Check sheet for the modelled part. Datum: model origin and axes. Units: mm. Face numbers are marked on the shaded views. Coordinates: 2 decimals unless noted, no trailing zeros. Write each loop counter-clockwise with the first axis right and the second up, starting at its lowest first coordinate (ties: lowest second). Pieces come first, ordered by that corner, then holes. Notation, with made-up numbers: (81.25, 41.25) - (110.25, 41.25) arc R23 ccw to (110.25, 68.25) - close; hole circle Ø2 at (70, 38). An arc over 180 degrees is marked (long way). Answer as CSV lines item,"result". Start each with the question number.
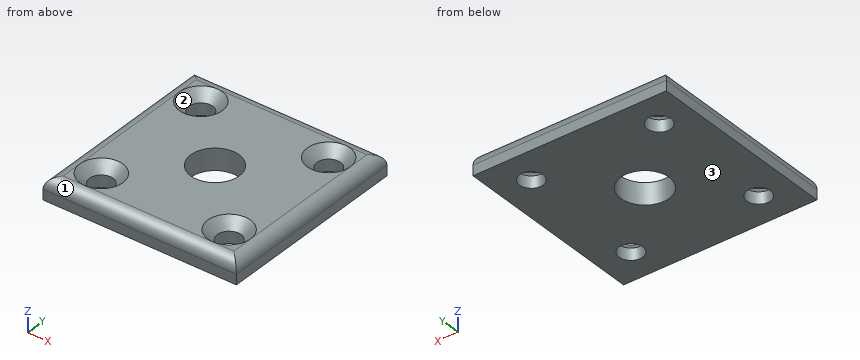
Autodesk Inventor part; units mm, degrees
ref_plane "YZ Plane" through (0, 0, 0) normal (1, 0, 0) x (0, 1, 0)
ref_plane "XZ Plane" through (0, 0, 0) normal (0, 1, 0) x (-1, 0, 0)
ref_plane "XY Plane" through (0, 0, 0) normal (0, 0, 1) x (1, 0, 0)
sketch "Эскиз1" plane through (0, 0, 0) normal (0, 0, 1) x (1, 0, 0)
  line L0 (0, 0) -> (18, 0)
  line L1 (18, 0) -> (18, 18)
  line L2 (18, 18) -> (0, 18)
  line L3 (0, 18) -> (0, 0)
  dimension "d0" = 18
  dimension "d1" = 18
extrude "Выдавливание1" add sketch "Эскиз1" along normal blind 2
sketch "Эскиз8" plane through (0, 0, 2) normal (0, 0, 1) x (1, 0, 0)
  line L0 (18, 18) -> (0, 18) construction
  line L1 (0, 0) -> (18, 18) construction
  line L2 (0, 0) -> (18, 0) construction
  line L3 (0, 18) -> (18, 0) construction
  circle A0 centre (9, 9) radius 2.25
  dimension "d38" = 4.5
extrude "Выдавливание5" cut sketch "Эскиз8" against normal through all
sketch "Эскиз9" plane through (0, 0, 2) normal (0, 0, 1) x (1, 0, 0)
  circle A0 centre (9, 9) radius 2.25 construction
  circle A1 centre (9, 9) radius 4.1 construction
  line L0 (0, 18) -> (0, 0) construction
  line L1 (0, 18) -> (6.1009, 11.8991) construction
  line L2 (18, 0) -> (18, 18) construction
  line L3 (18, 18) -> (11.8991, 11.8991) construction
  line L4 (0, 0) -> (6.1009, 6.1009) construction
  line L5 (0, 0) -> (18, 0) construction
  line L6 (18, 0) -> (11.8991, 6.1009) construction
  point P0 (3.0504, 14.9496)
  point P1 (14.9496, 14.9496)
  point P2 (3.0504, 3.0504)
  point P3 (14.9496, 3.0504)
  dimension "d41" = 8.2
hole "Отверстие4" at (3.0504, 14.9496, 2) at (3.0504, 3.0504, 2) at (14.9496, 3.0504, 2) at (14.9496, 14.9496, 2) direction (0, 0, -1) diameter 2.2 end through all countersink diameter 4 countersink angle 90
fillet "Сопряжение2" radius 1.05 4 edges at (9, 0, 2) (0, 9, 2) (9, 18, 2) (18, 9, 2)
properties part number "Крышка поворотного кулака"
(1) Cross-section at A-A on x = 9. Record the boundary of the cut face in (y, z), plus the area to 3 significant figures.
(2) Material ranges on probe 1 along Y at (x, z) = (14, 0.45); probe 2 along Y at (x, z) = (15.75, 0.75); probe 3 along X at (y, z) = (2.75, 0.45), recorded low to high. Write a range as from..to.
(3) Cross-section at C-C on z = 0.7. Record the boundary of the cut face in (x, y).
(4) Release check for a two-part mould opening along Y. For the marked faces 1, 2 and 3 record: pulls with the +Y half, pulls with the -Y half, needs draft (parallel to the pull), parting line crosses it, or undercut.
(5) Cross-section at D-D on y = 14.75. State how many separate pieces and enclosed holes the cut face has, plus the area to 3 significant figures.
Checked values:
1,outline,"(0, 0) - (6.75, 0) - (6.75, 2) - (1.05, 2) arc R1.05 ccw to (0, 0.95) - close; (11.25, 0) - (18, 0) - (18, 0.95) arc R1.05 ccw to (16.95, 2) - (11.25, 2) - close"
1,area,"26.5 mm^2"
2,probe 1,"0..2.5, 3.61..14.39, 15.5..18"
2,probe 2,"0..2.3, 3.8..14.2, 15.7..18"
2,probe 3,"0..1.99, 4.11..13.89, 16.01..18"
3,outline,"(0, 0) - (18, 0) - (18, 18) - (0, 18) - close; hole circle Ø2.2 at (3.05, 3.05); hole circle Ø2.2 at (3.05, 14.95); hole circle Ø4.5 at (9, 9); hole circle Ø2.2 at (14.95, 3.05); hole circle Ø2.2 at (14.95, 14.95)"
4,face 1,"pulls with the -Y half"
4,face 2,"undercut"
4,face 3,"needs draft"
5,separate pieces,"3"
5,enclosed holes,"0"
5,area,"25.2 mm^2"
